Autodesk Inventor part; units mm, degrees
ref_plane "Work Plane1" through (0, 15, 15) normal (0, 1, 0) x (-1, 0, 0)
ref_plane "YZ Plane" through (0, 0, 0) normal (1, 0, 0) x (0, 1, 0)
ref_plane "XZ Plane" through (0, 0, 0) normal (0, 1, 0) x (-1, 0, 0)
sketch "Sketch1" plane through (0, 0, 0) normal (0, 0, 1) x (1, 0, 0)
  circle A0 centre (0, 0) radius 2.15
  circle A1 centre (0, 0) radius 15
  dimension "d0" = 4.3
  dimension "d1" = 30
extrude "Extrusion1" add sketch "Sketch1" along normal blind 15
sketch "Sketch3" plane through (0, 0, 15) normal (0, 0, 1) x (1, 0, 0)
  point P0 (0, 0)
  point P1 (0, 15)
ref_plane "Work Plane1" through (0, 15, 15) normal (0, 1, 0) x (-1, 0, 0)
sketch "Sketch4" plane through (0, 15, 15) normal (0, 1, 0) x (-1, 0, 0)
  line L0 (15, 0) -> (-15, 0)
  line L1 (0, 0) -> (1.5987, 1.2017)
  line L2 (1.5987, 1.2017) -> (7.6071, -6.792)
  line L3 (7.6071, -6.792) -> (6.0084, -7.9937)
  line L4 (6.0084, -7.9937) -> (0, 0)
  line L5 (3.1858, -7.1278) -> (4.7814, -8.3336)
  line L6 (4.7814, -8.3336) -> (-1.2479, -16.3116)
  line L7 (-1.2479, -16.3116) -> (-2.8435, -15.1057)
  line L8 (-2.8435, -15.1057) -> (3.1858, -7.1278)
  point P0 (0, -15)
  dimension "d8" = 2
  dimension "d9" = 10
  dimension "d10" = 2
  dimension "d11" = 10
extrude "Extrusion3" cut sketch "Sketch4" against normal blind 3
pattern_circular "Circular Pattern1" count 8 over 360 about axis through (0, 0, 0) along (0, 0, 1) of "Extrusion3"
properties part number "Wheel"
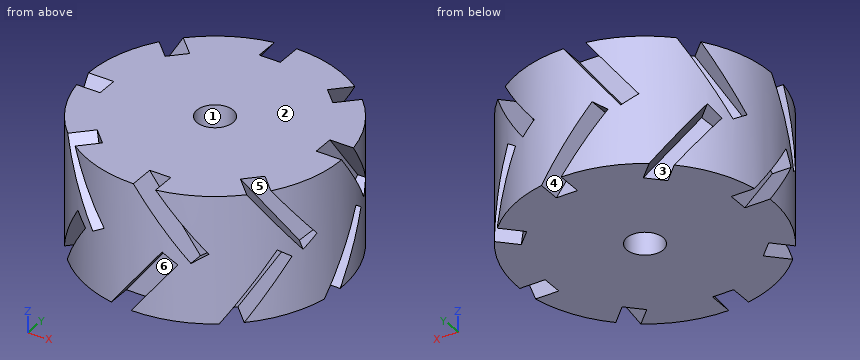
Geometry check sheet. Reference: the model listing, model coordinates, mm. Face numbers are marked on the shaded views. A direction names the side the tool comes from. Round coordinates to 2 decimals unless told otherwise and drop trailing zeros. Loops run counter-clockwise (first coordinate to the right, second up) from the corner with the lowest first, then second, coordinate; pieces in that order, holes last. Notation, with made-up numbers: (88.5, 58.5) - (93.5, 58.5) arc R11 cw to (93.5, 71.5) - close; hole circle Ø11 at (18.25, 69.25). An arc over 180 degrees is marked (long way). Write item = value, one per line. Start each with the question number.
1. Depth check by flat-ended pin: pin 1 (1 mm diameter, centred on y = -8, z = 1.5, fed in from -X); pin 2 (5 mm diameter, centred on x = 10, z = 3, fed in from +Y); pin 3 (2.5 mm diameter, centred on x = -1.5, z = 4.5, fed in from +Y). Enter the tip coordinate at first touch or a pass-through.
2. Section check C-C on y = -11.5. Enter the section's corners in (x, z).
3. Set-up check for the marked faces 4, 5 and 6: record each of +Z, -Z, +X, -X, +Y, -Y from which the full face is reachable in a straight line by a thin tool's end or side.
4. Thickness scan on line 1 (Y direction, x = 0, z = 10.25); line 2 (X direction, y = -5, z = 11); line 3 (Y direction, x = 8.25, z = 3). Record the ranges inside material, lowest first.
5. Section check A-A on y = 9.5. Enter the section's corners in (x, z), then the cut area to 3 significant figures.
6. Mould release check, pull along Z, two halves, no side actions. Record for the marked faces 1, 2 and 3: released by +Z, released by -Z, zero draft, split by the parting line, or undercut.
Working result:
q1.pin_1 = -12.99
q1.pin_2 = 12.99
q1.pin_3 = 15
q2.outline = (-9.63, 0) - (7.59, 0) - (9.63, 1.91) - (9.63, 15) - (-7.96, 15) - (-5.47, 12.66) - (-5.47, 9.33) - (-9.63, 13.24) - (-9.63, 5.41) - (-6.99, 7.87) - (-5.47, 7.06) - (-5.47, 5.98) - (-9.63, 2.09) - close
q3.face_4 = +Y
q3.face_5 = none
q3.face_6 = -Y
q4.line_1 = -15 to -2.15, 2.15 to 15
q4.line_2 = -12 to 11.97, 12.79 to 14.14
q4.line_3 = -12.53 to -8.95, -8.72 to 8.72, 11.09 to 12.53
q5.outline = (-11.61, 0) - (-9.14, 0) - (-11.61, 2.31) - close; (-11.61, 5.63) - (-7.47, 1.76) - (-7.47, 0) - (9.86, 0) - (7.47, 2.24) - (7.47, 5.56) - (11.61, 1.68) - (11.61, 15) - (9.5, 15) - (7.47, 13.09) - (7.47, 15) - (-9.5, 15) - (-11.61, 13.02) - close
q5.area = 319 mm^2
q6.face_1 = zero draft
q6.face_2 = released by +Z
q6.face_3 = undercut
